from build123d import *

# Parameters (mm, degrees)
SKETCH1_W           = 33
SKETCH1_H           = 35
BOSS_EXTRUDE1_DEPTH = 8
SKETCH2_W           = 20
SKETCH2_H           = 33
CUT_EXTRUDE1_DEPTH  = 7
CUT_EXTRUDE3_DEPTH  = 9
SKETCH3_W           = 14
SKETCH3_H           = 7
CUT_EXTRUDE4_DEPTH  = 7


with BuildPart() as part:
    # Sketch1 → Boss-Extrude1 (new body)
    with BuildSketch(Plane(origin=(0, 0, 0), x_dir=(1, 0, 0), z_dir=(0, 1, 0))):
        Rectangle(SKETCH1_W, SKETCH1_H)
    extrude(amount=BOSS_EXTRUDE1_DEPTH)

    # Sketch2 → Cut-Extrude1 (cut)
    with BuildSketch(Plane.XZ):
        Rectangle(SKETCH2_W, SKETCH2_H)
    extrude(amount=-CUT_EXTRUDE1_DEPTH, mode=Mode.SUBTRACT)

    # Sketch4 → Cut-Extrude3 (cut, through all)
    with BuildSketch(Plane(origin=(0, 8, 0), x_dir=(1, 0, 0), z_dir=(0, 1, 0))):
        with BuildLine():
            Line((14.5, 10.5), (14.5, -10.5))
            ThreePointArc((14.5, -10.5), (13, -12), (11.5, -10.5))
            Line((11.5, -10.5), (11.5, 10.5))
            ThreePointArc((11.5, 10.5), (13, 12), (14.5, 10.5))
        make_face()
        with BuildLine():
            Line((-14.5, 10.5), (-14.5, -10.5))
            ThreePointArc((-14.5, -10.5), (-13, -12), (-11.5, -10.5))
            Line((-11.5, -10.5), (-11.5, 10.5))
            ThreePointArc((-11.5, 10.5), (-13, 12), (-14.5, 10.5))
        make_face()
    extrude(amount=-CUT_EXTRUDE3_DEPTH, mode=Mode.SUBTRACT)

    # Sketch3 → Cut-Extrude4 (cut)
    with BuildSketch(Plane.XY.offset(17.5)):
        with Locations((0, 3.5)):
            Rectangle(SKETCH3_W, SKETCH3_H)
    extrude(amount=-CUT_EXTRUDE4_DEPTH, mode=Mode.SUBTRACT)


solid = part.part
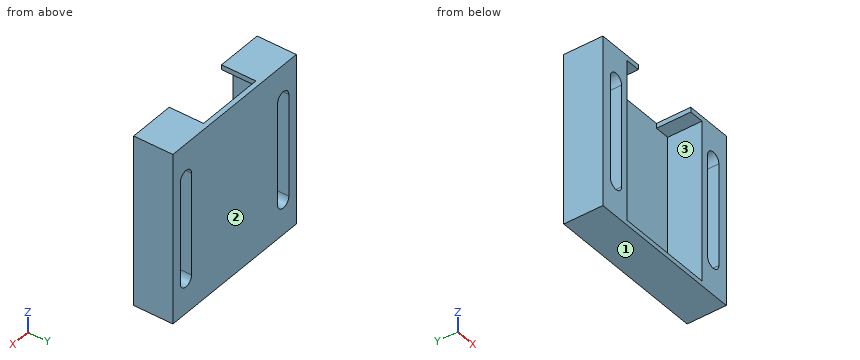
Build history of the part. All positions in model axes, mm. Face numbers are marked on the shaded views. Give positions to 0.01 mm unless a question says otherwise; leave off trailing zeros. Order: outer loops, then holes, each group sorted by start corner. A loop starts at its lowest first (then second) coordinate and runs counter-clockwise, first axis right, second up. Notation, with made-up numbers: M 75.5,-26.5 L 85.5,-26.5 A26 ccw 85.5,-1.5 Z; hole C 39,5 d3. An arc over 180 degrees is marked long. Put each result on its own line as item: value.
Item 1: Cut at D-D on z = -14. Write the cut outline in (x, y).
Results are:
outline: M -16.5,0 L -10,0 L -10,7 L 10,7 L 10,0 L 16.5,0 L 16.5,8 L -16.5,8 Z
Item 2: Wall check: probe 1 along X at (y, z) = (0.75, -8); probe 2 along X at (y, z) = (7.25, -8); probe 3 along X at (y, z) = (4, -12.5). Give the ranges that are in metal, low to high.
Results are:
probe 1: -16.5 to -14.5, -11.5 to -10, 10 to 11.5, 14.5 to 16.5
probe 2: -16.5 to -14.5, -11.5 to 11.5, 14.5 to 16.5
probe 3: -16.5 to -10, 10 to 16.5
Item 3: Cut at C-C on x = 13. Write the cut outline in (y, z), then the cut area to 3 significant figures.
Results are:
outline: M 0,-17.5 L 8,-17.5 L 8,-12 L 0,-12 Z; M 0,12 L 8,12 L 8,17.5 L 0,17.5 Z
area: 88.0 mm2
Item 4: Cut at B-B on y = 6.5. Write the cut outline in (x, z), then the cut area to 3 significant figures.
Results are:
outline: M -16.5,-17.5 L 16.5,-17.5 L 16.5,17.5 L 7,17.5 L 7,16.5 L 10,16.5 L 10,-16.5 L -10,-16.5 L -10,16.5 L -7,16.5 L -7,17.5 L -16.5,17.5 Z; hole M -14.5,-10.5 A1.5 ccw -11.5,-10.5 L -11.5,10.5 A1.5 ccw -14.5,10.5 Z; hole M 11.5,-10.5 A1.5 ccw 14.5,-10.5 L 14.5,10.5 A1.5 ccw 11.5,10.5 Z
area: 341 mm2
Item 5: Cut at A-A on z = 4.5. Write the cut outline in (x, y), then the cut area to 3 significant figures.
Results are:
outline: M -16.5,0 L -14.5,0 L -14.5,8 L -16.5,8 Z; M -11.5,0 L -10,0 L -10,7 L 10,7 L 10,0 L 11.5,0 L 11.5,8 L -11.5,8 Z; M 14.5,0 L 16.5,0 L 16.5,8 L 14.5,8 Z
area: 76.0 mm2
Item 6: Pull direction Z, two halves, no side cores. Call the marked faces 1, 2 and 3: +Z half, -Z half, draft (parallel to the pull), parting line (faces both ways), or undercut.
Results are:
face 1: -Z half
face 2: draft
face 3: undercut
Item 7: Drop flat-ended pins along their axis: pin 1 Ø3.5 at (x, y) = (4, 3) entering from +Z; pin 2 Ø6 at (x, z) = (-3.5, 0) entering from -Y. Give the stop position or say it passes through.
Results are:
pin 1: z = -16.5
pin 2: y = 7
